Model file for the job. Use its own axes, mm. Face numbers are marked on the shaded views. A direction names the side the tool comes from. Round coordinates to 2 decimals unless told otherwise and drop trailing zeros. Order: outer loops, then holes, each group sorted by start corner. A loop starts at its lowest first (then second) coordinate and runs counter-clockwise, first axis right, second up. Notation, with made-up numbers: (3.25, 71.5) - (28.25, 71.5) arc R21 ccw to (28.25, 103.5) - close; hole circle Ø3 at (70, -33). An arc over 180 degrees is marked (long way). Write item = value, one per line.
```python
from build123d import *

# Parameters (mm, degrees)
SKETCH1_R           = 17.5
SKETCH1_R_2         = 11
BOSS_EXTRUDE1_DEPTH = 3.5
SKETCH4_R           = 4
CUT_EXTRUDE1_DEPTH  = 6.5
CIRPATTERN1_COUNT   = 8


with BuildPart() as part:
    # Sketch1 → Boss-Extrude1 (new body, symmetric)
    with BuildSketch(Plane.XY):
        Circle(SKETCH1_R)
        Circle(SKETCH1_R_2, mode=Mode.SUBTRACT)
    extrude(amount=BOSS_EXTRUDE1_DEPTH, both=True)

    # Sketch4 → Cut-Extrude1 (cut)
    with BuildSketch(Plane(origin=(-10.162674858, 0, 0), x_dir=(0, 0, -1), z_dir=(1, 0, 0))):
        Circle(SKETCH4_R)
    cut_extrude1 = extrude(amount=-CUT_EXTRUDE1_DEPTH, mode=Mode.SUBTRACT)

    # CirPattern1: Cut-Extrude1 ×8 about axis
    cirpattern1_axis = Axis((0, 0, 0), (0, 0, 1))
    for i in range(1, CIRPATTERN1_COUNT):
        add(cut_extrude1.rotate(cirpattern1_axis, i * 360 / CIRPATTERN1_COUNT), mode=Mode.SUBTRACT)


solid = part.part
```
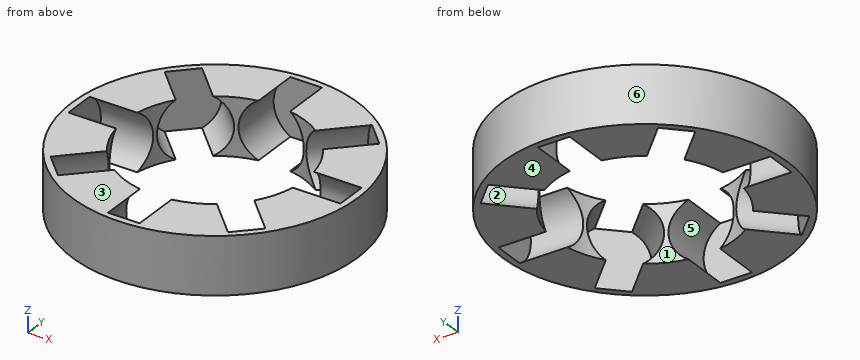
1) Flat gauge pins, fed straight in: pin 1 Ø2 at (y, z) = (-2, -0.5) entering from -X; pin 2 Ø1.5 at (y, z) = (-9, 2.5) entering from -X; pin 3 Ø4 at (x, z) = (-13.5, -0.5) entering from -Y. Where does each tip first touch, or does it go through?
Conclusion:
pin_1 = -17.47
pin_2 = -15.43
pin_3 = -13.19
2) Mould opens along Y. For the marked faces 4, 5 and 6 say: +Y half, -Y half, draft (parallel to the pull), parting line (faces both ways), or undercut.
Conclusion:
face_4 = draft
face_5 = undercut
face_6 = parting line
3) 3-axis set-ups, long thin cutter, end or side, ignore diameter. For the marked faces 1, 2 and 3: which of +Z, -Z, +X, -X, +Y, -Y reach the whole face in a straight line?
Conclusion:
face_1 = +Z, -Z
face_2 = none
face_3 = +Z, +X, -X, +Y, -Y
4) Wall check: line 1 along Y through (x, z) = (11.5, -2.75); line 2 along Y through (x, z) = (11, -3); line 3 along X through (y, z) = (11.5, 1). Give the ranges that are in metal, low to high.
Conclusion:
line_1 = -13.19 to -12.06, -7.39 to -2.9, 2.9 to 7.39, 12.06 to 13.19
line_2 = -13.61 to -12.56, -7.26 to -2.65, 2.65 to 7.26, 12.56 to 13.61
line_3 = -13.19 to -12.06, -6.02 to -3.87, 3.87 to 6.02, 12.06 to 13.19
5) Cut at A-A (y = 0). Write the cut outline in (x, z), and give its area (3 significant figures).
Conclusion:
outline = (-17.5, -3.5) - (-16.66, -3.5) - (-16.66, 3.5) - (-17.5, 3.5) - close; (16.66, -3.5) - (17.5, -3.5) - (17.5, 3.5) - (16.66, 3.5) - close
area = 11.7 mm^2
6) Cut at D-D (y = 9.5). Give the number of separate pieces and of enclosed holes in the cut face, and give its area (3 significant figures).
Conclusion:
separate_pieces = 6
enclosed_holes = 0
area = 13.8 mm^2
